```python
from build123d import *

# Parameters (mm, degrees)
SKETCH1_W                                    = 40
SKETCH1_H                                    = 10
BOSS_EXTRUDE1_DEPTH                          = 3
CSK_FOR_M3_COUNTERSUNK_FLAT_HEAD_SCR_2_COUNT = 2
CSK_FOR_M3_COUNTERSUNK_FLAT_HEAD_SCR_2_PITCH = 28
CSK_FOR_M3_COUNTERSUNK_FLAT_HEAD_SCR_3_COUNT = 2
CSK_FOR_M3_COUNTERSUNK_FLAT_HEAD_SCR_3_PITCH = 14


with BuildPart() as part:
    # Sketch1 → Boss-Extrude1 (new body)
    with BuildSketch(Plane(origin=(0, 0, 0), x_dir=(1, 0, 0), z_dir=(0, 1, 0))):
        Rectangle(SKETCH1_W, SKETCH1_H)
    extrude(amount=BOSS_EXTRUDE1_DEPTH)

    # Sketch3 → CSK for M3 Countersunk Flat Head Screw1 (revolve, cut)
    with BuildSketch(Plane(origin=(-14, 3, 0), x_dir=(0, 0, 1), z_dir=(1, 0, 0))):
        Polygon((0, 0), (0, 3), (1.7, 3), (1.7, 1.45), (3.15, 0), align=None)
    csk_for_m3_countersunk_flat_head_screw1 = revolve(axis=Axis((-14, 9.35, 0), (0, -1, 0)), mode=Mode.SUBTRACT)

    # CSK for M3 Countersunk Flat Head Scr 2: CSK for M3 Countersunk Flat Head Screw1 ×2
    with Locations(*[(i * CSK_FOR_M3_COUNTERSUNK_FLAT_HEAD_SCR_2_PITCH, 0, 0) for i in range(1, CSK_FOR_M3_COUNTERSUNK_FLAT_HEAD_SCR_2_COUNT)]):
        add(csk_for_m3_countersunk_flat_head_screw1, mode=Mode.SUBTRACT)

    # CSK for M3 Countersunk Flat Head Scr 3: CSK for M3 Countersunk Flat Head Screw1 ×2
    with Locations(*[(i * CSK_FOR_M3_COUNTERSUNK_FLAT_HEAD_SCR_3_PITCH, 0, 0) for i in range(1, CSK_FOR_M3_COUNTERSUNK_FLAT_HEAD_SCR_3_COUNT)]):
        add(csk_for_m3_countersunk_flat_head_screw1, mode=Mode.SUBTRACT)


solid = part.part
```
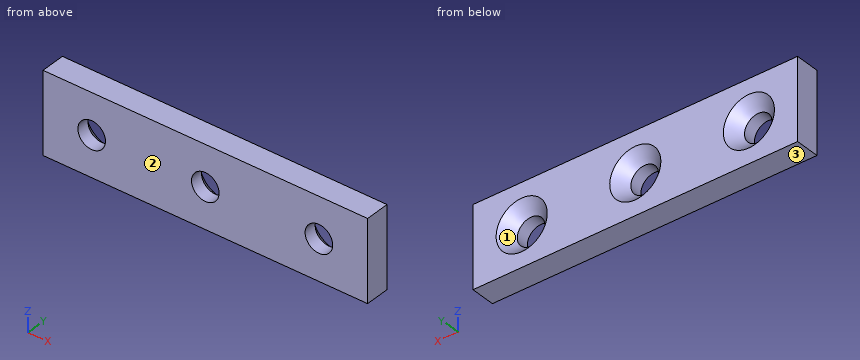
Read the model definition and answer for the solid it produces. Units are mm, in the model's axes. Face numbers are marked on the shaded views. Round coordinates to 2 decimals unless told otherwise and drop trailing zeros. Write each loop counter-clockwise with the first axis right and the second up, starting at its lowest first coordinate (ties: lowest second). Pieces come first, ordered by that corner, then holes. Notation, with made-up numbers: M 21.5,40.25 L 32.5,40.25 A14 cw 32.5,51.25 Z; hole C -29,63.25 d4. An arc over 180 degrees is marked long. One line per item, written item: value.
Q1. Straight lines are drawn through the part: line 1 (X direction, y = 0.85, z = 0); line 2 (X direction, y = 2.1, z = 0.5); line 3 (Z direction, x = 14, y = 1.05). For each, find the intervals that lie inside material, in ascending order. Write a range as [from, to].
Data:
line 1: [-20, -15.7], [-12.3, -1.7], [1.7, 12.3], [15.7, 20]
line 2: [-20, -16.19], [-11.81, -2.19], [2.19, 11.81], [16.19, 20]
line 3: [-5, -1.7], [1.7, 5]
Q2. Find section C-C on y = 2.45. Write down the section's boundary in (x, z), plus the area to 3 significant figures.
Data:
outline: M -20,-5 L 20,-5 L 20,5 L -20,5 Z; hole C -14,0 d5.2; hole C 0,0 d5.2; hole C 14,0 d5.2
area: 336 mm2
Q3. For a pull along Z with two mould halves and no side action, classify the marked faces 1, 2 and 3 as +Z half, -Z half, draft (parallel to the pull), parting line (faces both ways), or undercut.
Data:
face 1: undercut
face 2: draft
face 3: -Z half
Q4. Find section A-A on x = -14. Write down the section's boundary in (y, z).
Data:
outline: M 0,-5 L 3,-5 L 3,-3.15 L 1.55,-1.7 L 0,-1.7 Z; M 0,1.7 L 1.55,1.7 L 3,3.15 L 3,5 L 0,5 Z
Q5. Find section B-B on z = 0. Write down the section's boundary in (x, y), plus the area to 3 significant figures.
Data:
outline: M -20,0 L -15.7,0 L -15.7,1.55 L -17.15,3 L -20,3 Z; M -12.3,0 L -1.7,0 L -1.7,1.55 L -3.15,3 L -10.85,3 L -12.3,1.55 Z; M 1.7,0 L 12.3,0 L 12.3,1.55 L 10.85,3 L 3.15,3 L 1.7,1.55 Z; M 15.7,0 L 20,0 L 20,3 L 17.15,3 L 15.7,1.55 Z
area: 83.1 mm2
Q6. Flat-ended cylindrical pins translate along their axes: pin 1 Ø4 at (x, z) = (14, 0) entering from +Y; pin 2 Ø5.5 at (x, z) = (-14, 0) entering from +Y. Find the tip coordinate at first contact, or state that the pin passes through.
Data:
pin 1: y = 1.85
pin 2: y = 2.6
